from build123d import *

# Parameters (mm, degrees)
ESQUISSE1_W             = 200
ESQUISSE1_H             = 74
BOSS_EXTRU_1_DEPTH      = 6.35
ESQUISSE2_W             = 6.35
ESQUISSE2_H             = 10.571428571
ENL_V_MAT_EXTRU_1_DEPTH = 6.35
ESQUISSE3_W             = 18.181818182
ESQUISSE3_H             = 6.35
ESQUISSE3_W_2           = 18.181818181
ENL_V_MAT_EXTRU_2_DEPTH = 6.35


with BuildPart() as part:
    # Esquisse1 → Boss.-Extru.1 (new body)
    with BuildSketch(Plane(origin=(0, 0, 0), x_dir=(1, 0, 0), z_dir=(0, 1, 0))):
        with Locations((0, 37)):
            Rectangle(ESQUISSE1_W, ESQUISSE1_H)
    extrude(amount=BOSS_EXTRU_1_DEPTH)

    # Esquisse2 → Enlèv. mat.-Extru.1 (cut)
    with BuildSketch(Plane(origin=(0, 6.35, 0), x_dir=(1, 0, 0), z_dir=(0, 1, 0))):
        with Locations((96.825, 68.714285714)):
            Rectangle(ESQUISSE2_W, ESQUISSE2_H)
        with Locations((96.825, 47.571428572)):
            Rectangle(ESQUISSE2_W, ESQUISSE2_H)
        with Locations((96.825, 26.428571428)):
            Rectangle(ESQUISSE2_W, ESQUISSE2_H)
        with Locations((96.825, 5.285714286)):
            Rectangle(ESQUISSE2_W, ESQUISSE2_H)
    enl_v_mat_extru_1 = extrude(amount=-ENL_V_MAT_EXTRU_1_DEPTH, mode=Mode.SUBTRACT)

    # Symétrie1: Enlèv. mat.-Extru.1 across plane
    add(enl_v_mat_extru_1.mirror(Plane(origin=(0, 0, 0), x_dir=(0, 0, 1), z_dir=(1, 0, 0))), mode=Mode.SUBTRACT)

    # Esquisse3 → Enlèv. mat.-Extru.2 (cut)
    with BuildSketch(Plane(origin=(0, 6.35, 0), x_dir=(1, 0, 0), z_dir=(0, 1, 0))):
        with Locations((-90.909090909, 70.825)):
            Rectangle(ESQUISSE3_W, ESQUISSE3_H)
        with Locations((-54.545454546, 70.825)):
            Rectangle(ESQUISSE3_W_2, ESQUISSE3_H)
        with Locations((-18.181818182, 70.825)):
            Rectangle(ESQUISSE3_W, ESQUISSE3_H)
        with Locations((18.181818182, 70.825)):
            Rectangle(ESQUISSE3_W, ESQUISSE3_H)
        with Locations((54.545454546, 70.825)):
            Rectangle(ESQUISSE3_W_2, ESQUISSE3_H)
        with Locations((90.909090909, 70.825)):
            Rectangle(ESQUISSE3_W, ESQUISSE3_H)
    extrude(amount=-ENL_V_MAT_EXTRU_2_DEPTH, mode=Mode.SUBTRACT)


solid = part.part
Build history of the part. All positions in model axes, mm. A direction names the side the tool comes from. Round coordinates to 2 decimals unless told otherwise and drop trailing zeros. Write each loop counter-clockwise with the first axis right and the second up, starting at its lowest first coordinate (ties: lowest second). Pieces come first, ordered by that corner, then holes. Notation, with made-up numbers: (-29, 31.25) - (-9, 31.25) arc R22 cw to (-9, 43.25) - close; hole circle Ø10 at (35.25, 88). An arc over 180 degrees is marked (long way). One line per question, with ' | ' between items.
1. Band-saw the part on A-A, the plane x = -54.5. Write the cut outline in (y, z).
Results are:
outline: (0, -67.65) - (6.35, -67.65) - (6.35, 0) - (0, 0) - close
2. Drop flat-ended pins along their axis: pin 1 Ø3 at (y, z) = (3.5, -69.5) entering from +X; pin 2 Ø1.9 at (x, y) = (-96.5, 4) entering from -Z; pin 3 Ø3 at (y, z) = (3.5, -71) entering from -X. Give the stop position or say it passes through.
Results are:
pin 1: x = 81.82 | pin 2: z = -63.43 | pin 3: x = -81.82
3. Mould opens along X. For faces 1 (the face through (-93.65, 3, -26)), 2 (the face through (36, 3, -74)), 3 (the face through (-27.273, 3, -71)), 4 (the face through (81.818, 3, -71)) say: released by +X, released by -X, zero draft, split by the parting line, or undercut.
Results are:
face 1: released by -X | face 2: zero draft | face 3: undercut | face 4: released by +X
4. Band-saw the part on B-B, the plane z = -24. Write the cut outline in (x, y).
Results are:
outline: (-93.65, 0) - (93.65, 0) - (93.65, 6.35) - (-93.65, 6.35) - close
5. Drill centre lines: line 1 along Z through (x, y) = (21.5, 5); line 2 along X through (y, z) = (1.25, -26). Where is each one in solid material? Low to high. Write a range as from..to.
Results are:
line 1: -67.65..0 | line 2: -93.65..93.65
6. Tool access for faces 5 (the face through (-93.65, 3, -5)), 6 (the face through (-97, 3, -63.429)), 7 (the face through (-45.455, 3, -71)), 8 (the face through (-97, 3, -31.714)): list every direction of +Z, -Z, +X, -X, +Y, -Y with a clear straight run to the whole face (end or side of a thin tool).
Results are:
face 5: +Z, -X, +Y, -Y | face 6: -Z, -X, +Y, -Y | face 7: -Z, +Y, -Y | face 8: -X, +Y, -Y
